from build123d import *


with BuildPart() as part:
    # Sketch1 → Revolve1 (revolve)
    with BuildSketch(Plane(origin=(0, 0, 0), x_dir=(0, 0, -1), z_dir=(1, 0, 0)), mode=Mode.PRIVATE) as revolve1_sk:
        with BuildLine():
            Line((-4, 7.45), (-2.236067977, 7.45))
            ThreePointArc((-2.236067977, 7.45), (0, 6.45), (2.236067977, 7.45))
            Line((2.236067977, 7.45), (4, 7.45))
            Line((4, 7.45), (4, 5.25))
            ThreePointArc((4, 5.25), (3.912132034, 5.037867966), (3.7, 4.95))
            Line((3.7, 4.95), (-3.7, 4.95))
            ThreePointArc((-3.7, 4.95), (-3.912132034, 5.037867966), (-4, 5.25))
            Line((-4, 5.25), (-4, 7.45))
        make_face()
    revolve(revolve1_sk.sketch.rotate(Axis((0, 0, 7.419354839), (0, 0, -1)), 90), axis=Axis((0, 0, 7.419354839), (0, 0, -1)))


solid = part.part
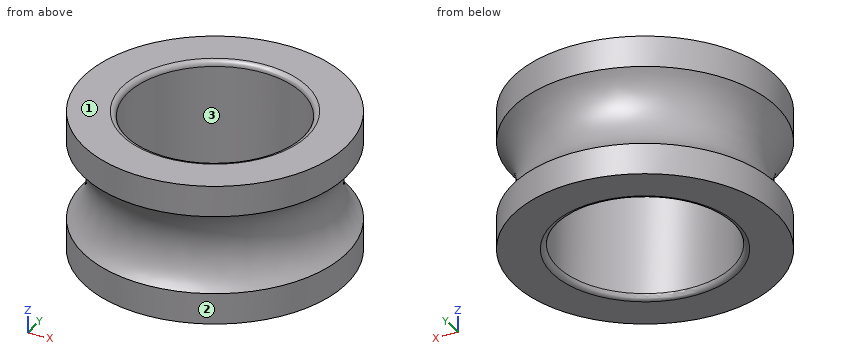
Part model, mm, in its own coordinate system. Face numbers are marked on the shaded views. Coordinates: 2 decimals unless noted, no trailing zeros. Loops run counter-clockwise (first coordinate to the right, second up) from the corner with the lowest first, then second, coordinate; pieces in that order, holes last. Notation, with made-up numbers: M 60.25,-20 L 96.25,-20 A26 ccw 96.25,1 Z; hole C -2,56 d6. An arc over 180 degrees is marked long. Use a Markdown table: item, result. Add a question column.
Q1. Pin check, flat tips, straight feed: P1, Ø4, axis at y = 5.5, z = -0.5, coming from the +X side; P2, Ø1.5, axis at y = -2, z = -3, coming from the -X side; P3, Ø4, axis at y = 5.5, z = 1.5, coming from the -X side. Stop position of each tip, or through.
Q2. Cut at C-C (z = 0). Write the cut outline in (x, y).
Q3. Cut at D-D (z = 3). Write the cut outline in (x, y).
Q4. Cut at A-A (y = 0). Write the cut outline in (x, z), and give its area (3 significant figures).
Q5. Mould opens along Y. For the marked faces 1, 2 and 3 say: +Y half, -Y half, draft (parallel to the pull), parting line (faces both ways), or undercut.
Q6. Probe L1, parallel to Z at x = -6.5, y = 2; L2, parallel to Z at x = -6.5, y = 3.5; L3, parallel to X at y = -1.5, z = 0. List the from-to ranges inside material, lowest first.
Worked out:
| question | item | result |
|---|---|---|
| 1 | P1 | stops at x = 5.93 |
| 1 | P2 | stops at x = -7.34 |
| 1 | P3 | stops at x = -6.5 |
| 2 | outline | C 0,0 d12.9; hole C 0,0 d9.9 |
| 3 | outline | C 0,0 d14.9; hole C 0,0 d9.9 |
| 4 | outline | M -7.45,-4 L -5.25,-4 A0.3 ccw -4.95,-3.7 L -4.95,3.7 A0.3 ccw -5.25,4 L -7.45,4 L -7.45,2.24 A3 cw -7.45,-2.24 Z; M 4.95,-3.7 A0.3 ccw 5.25,-4 L 7.45,-4 L 7.45,-2.24 A3 cw 7.45,2.24 L 7.45,4 L 5.25,4 A0.3 ccw 4.95,3.7 Z |
| 4 | area | 33.7 mm2 |
| 5 | face 1 | draft |
| 5 | face 2 | parting line |
| 5 | face 3 | undercut |
| 6 | L1 | z = -4 to -1.41, 1.41 to 4 |
| 6 | L2 | z = -4 to -2.17, 2.17 to 4 |
| 6 | L3 | x = -6.27 to -4.72, 4.72 to 6.27 |
